Verification items for this drawing (mm, ordinates from the low corner). A direction names the side the tool comes from. Give positions to 0.01 mm unless a question says otherwise; leave off trailing zeros. Loops run counter-clockwise (first coordinate to the right, second up) from the corner with the lowest first, then second, coordinate; pieces in that order, holes last. Notation, with made-up numbers: (-0.75, 40.5) -> (33.25, 40.5) arc R21 cw to (33.25, 65.5) -> close; hole circle Ø9 at (5, 59.25). An arc over 180 degrees is marked (long way). Write item = value, one per line.
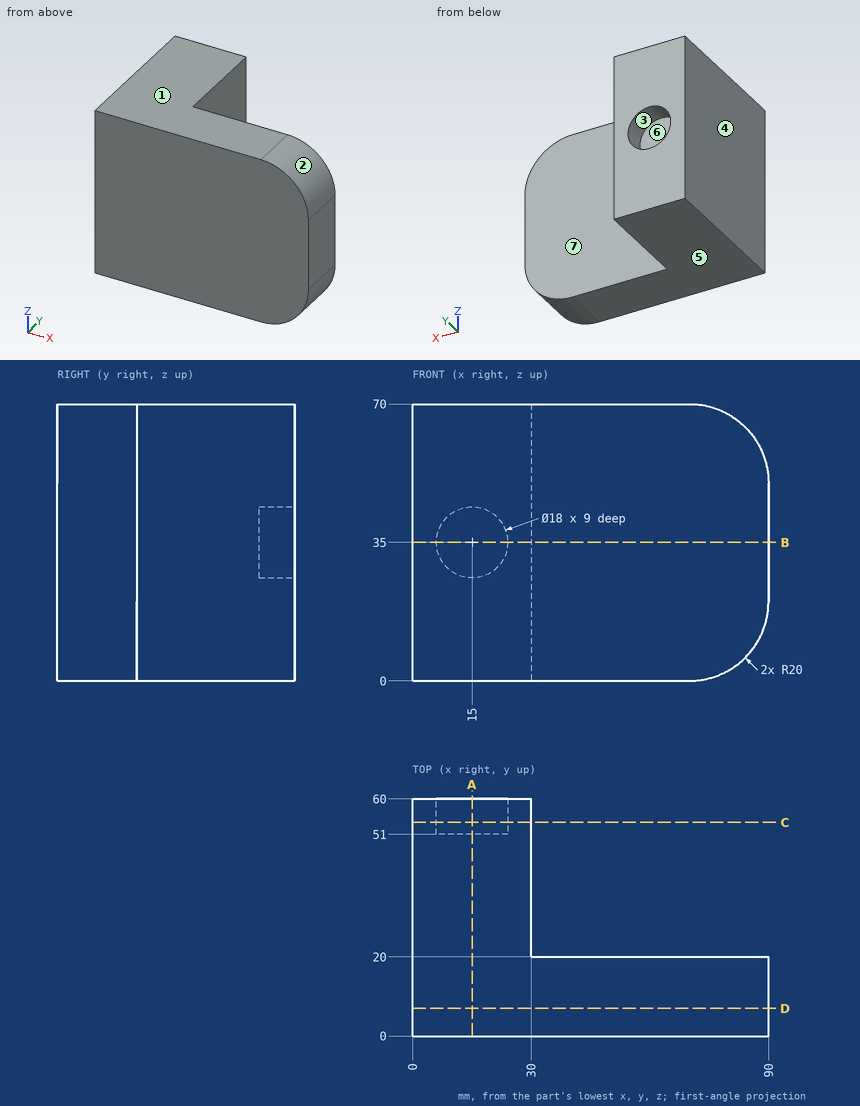
Item 1: Section check B-B, the plane z = 35. Record the cut outline in (x, y).
Answer:
outline = (0, 0) -> (90, 0) -> (90, 20) -> (30, 20) -> (30, 60) -> (24, 60) -> (24, 51) -> (6, 51) -> (6, 60) -> (0, 60) -> close
Item 2: Thickness scan on L1, parallel to X at y = 53.25, z = 35; L2, parallel to Z at x = 15, y = 57.5; L3, parallel to Y at x = 61, z = 19. Record the ranges inside material, lowest first. Write a range as [from, to].
Answer:
L1 = [0, 6], [24, 30]
L2 = [0, 26], [44, 70]
L3 = [0, 20]
Item 3: Gauge pin test, flat ends, axial feed: pin 1 (5 mm diameter, centred on x = 25, z = 32, fed in from -Y); pin 2 (3 mm diameter, centred on x = 52, z = 56.5, fed in from +Y); pin 3 (12 mm diameter, centred on y = 36.5, z = 48, fed in from +X). Record the tip position at first contact, or that the pin passes through.
Answer:
pin_1 = 0
pin_2 = 20
pin_3 = 30
Item 4: Section check D-D, the plane y = 7. Record the cut outline in (x, z), plus the area to 3 significant figures.
Answer:
outline = (0, 0) -> (70, 0) arc R20 ccw to (90, 20) -> (90, 50) arc R20 ccw to (70, 70) -> (0, 70) -> close
area = 6,130 mm^2
Item 5: Tool access check on the marked faces 5, 6 and 7. Record the directions out of +Z, -Z, +X, -X, +Y, -Y that give a thin tool (end or side, any length) a straight path to the whole face; none if there is none.
Answer:
face_5 = -Z, +X, -X, +Y, -Y
face_6 = +Y
face_7 = +Z, -Z, +X, +Y
Item 6: Section check A-A, the plane x = 15. Record the cut outline in (y, z).
Answer:
outline = (0, 0) -> (60, 0) -> (60, 26) -> (51, 26) -> (51, 44) -> (60, 44) -> (60, 70) -> (0, 70) -> close
Item 7: Draft check along X on the marked faces 1, 2, 3 and 4. Enter one of: +X half, -X half, draft (parallel to the pull), parting line (faces both ways), or undercut.
Answer:
face_1 = draft
face_2 = +X half
face_3 = undercut
face_4 = -X half
Item 8: Section check C-C, the plane y = 54. Record the cut outline in (x, z), plus the area to 3 significant figures.
Answer:
outline = (0, 0) -> (30, 0) -> (30, 70) -> (0, 70) -> close; hole circle Ø18 at (15, 35)
area = 1,850 mm^2
